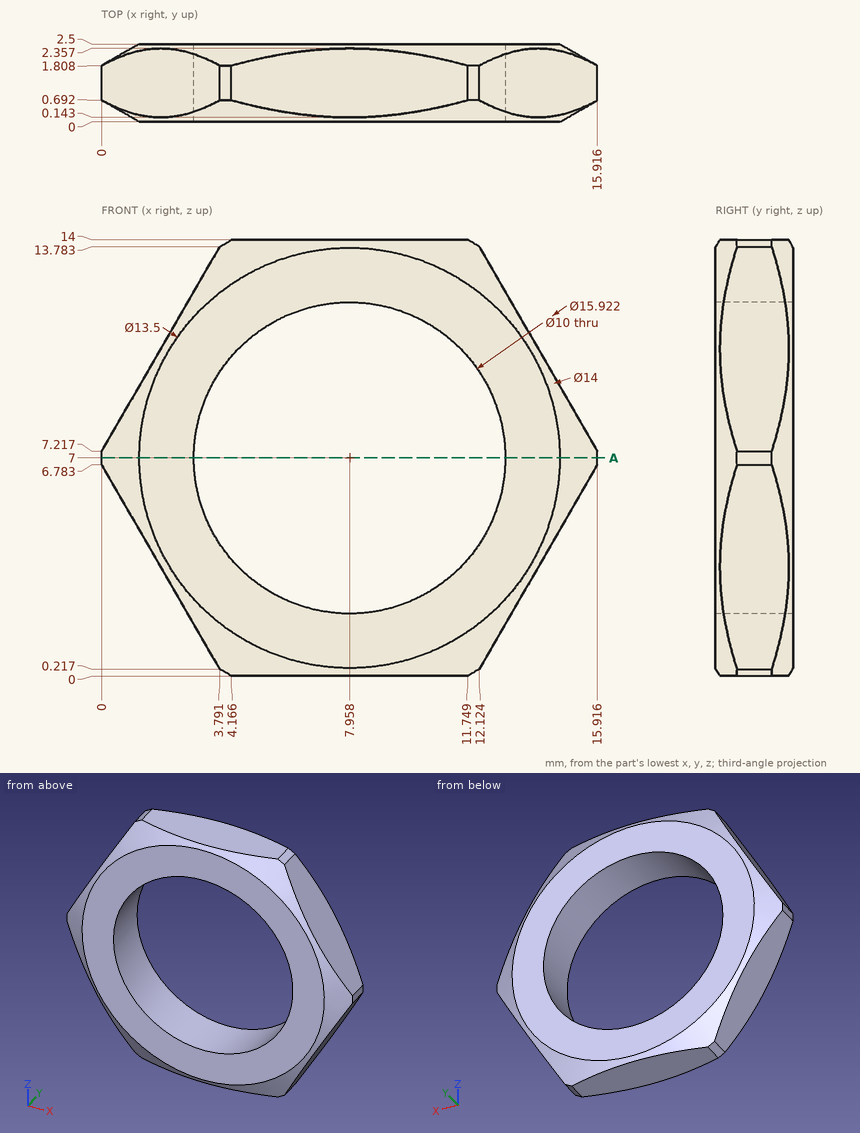
Geometry check sheet. Reference: drawing and pictorial views, mm from the part's lowest x, y, z. Give positions to 0.01 mm unless a question says otherwise; leave off trailing zeros. Order: outer loops, then holes, each group sorted by start corner. A loop starts at its lowest first (then second) coordinate and runs counter-clockwise, first axis right, second up. Notation, with made-up numbers: M 54.25,71.25 L 92.25,71.25 A17 cw 92.25,79.25 Z; hole C 5.5,53 d5. An arc over 180 degrees is marked long. Answer as a JSON object with one key per item and string values. Group by question number.
1) Cross-section at A-A (z = 7). Enter the section's corners in (x, y) (1 decimal).
2) Depth check by flat-ended pin: pin 1 Ø3 at (x, z) = (11, 10.5) entering from -Y; pin 2 Ø1.5 at (y, z) = (1, 12.5) entering from +X. Enter the tip coordinate at first touch or a pass-through.
3) Scan lines: line 1 along Z through (x, y) = (7.75, 1.05) (1 decimal); line 2 along X through (y, z) = (1.35, 7.75) (1 decimal); line 3 along X through (y, z) = (2.05, 6) (1 decimal). Record each from-to range of solid material in increasing order. Write a range as [from, to].
Result sheet:
{
 "1": {"outline": "M 0,0.7 L 1.2,0 L 3,0 L 3,2.5 L 1.2,2.5 L 0,1.8 Z; M 13,0 L 14.7,0 L 15.9,0.7 L 15.9,1.8 L 14.7,2.5 L 13,2.5 Z"},
 "2": {"pin 1": "stops at y = 0", "pin 2": "stops at x = 13.3"},
 "3": {"line 1": "z = [0, 2], [12, 14]", "line 2": "x = [0.3, 3], [12.9, 15.6]", "line 3": "x = [0.5, 3.1], [12.9, 15.4]"}
}
